Model file for the job. Use its own axes, mm. Face numbers are marked on the shaded views. A direction names the side the tool comes from. Coordinates: 2 decimals unless noted, no trailing zeros. Write each loop counter-clockwise with the first axis right and the second up, starting at its lowest first coordinate (ties: lowest second). Pieces come first, ordered by that corner, then holes. Notation, with made-up numbers: M 78.25,76.25 L 132.25,76.25 A21 cw 132.25,85.25 Z; hole C 59.25,-31.75 d10. An arc over 180 degrees is marked long. Put each result on its own line as item: value. Start each with the question number.
Q1. Cut at C-C (z = 14.5). Write the cut outline in (x, y), then the cut area to 3 significant figures.
Q2. Which spindle directions (+Z, -Z, +X, -X, +Y, -Y) get a long thin tool onto all of the face, cutting with end or side? Do the marked faces 1, 2 and 3. Say none if no direction does.
Q3. Pull direction Y, two halves, no side cores. Call the marked faces 4, 5 and 6: pulls with the +Y half, pulls with the -Y half, needs draft (parallel to the pull), parting line crosses it, or undercut.
Q4. Cut at A-A (z = 11). Write the cut outline in (x, y).
Q5. Drop flat-ended pins along their axis: pin 1 (10 mm diameter, centred on x = -7.5, z = 6, fed in from -Y); pin 2 (0.9 mm diameter, centred on x = 16.5, z = 0, fed in from -Y); pin 3 (12 mm diameter, centred on x = 31, z = 9, fed in from +Y); pin 4 (3 mm diameter, centred on x = 27.5, z = 10, fed in from -Y). Give the stop position or say it passes through.
Q6. Cut at B-B (x = 21.5). Give the number of separate pieces and of enclosed holes in the cut face, then the cut area to 3 significant figures.
Q7. Drill centre lines: line 1 along Y through (x, z) = (-1, 15.25); line 2 along Z through (x, y) = (33, -30); line 3 along Y through (x, z) = (0, 12). Where is each one in solid material? Low to high.
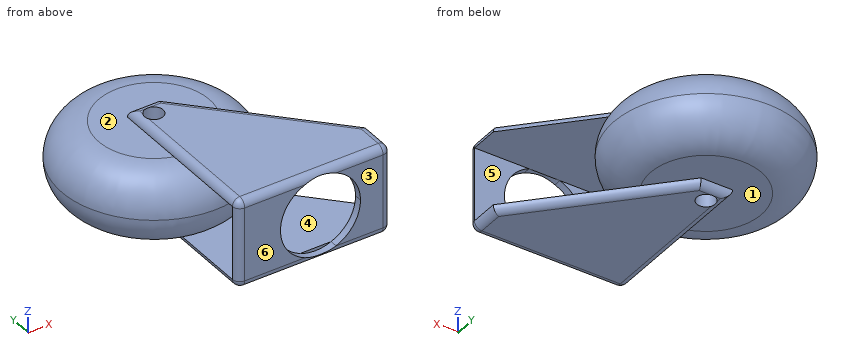
```python
from build123d import *

# Parameters (mm, degrees)
F0_R          = 25
F1_DEPTH      = 20
F2_R          = 9.99999
F3_R          = 2.5
F4_DEPTH      = 25.4
F5_R          = 2.5
F6_DEPTH      = 2
F7_W          = 41.5132804774
F7_H          = 2
F8_DEPTH      = 20
F9_R          = 2.5
F9_W          = 41.5132804774
F9_H          = 2
F10_DEPTH     = 2
F11_T1_DEPTH  = 20
F11_T3_DEPTH  = 47.4638193212
F11_T5_DEPTH  = 37.5132804774
F11_T7_DEPTH  = 12.6040666103
F11_T9_DEPTH  = 57.9730332998
F11_T11_DEPTH = 18.5555869155
F11_T13_DEPTH = 57.9730332998
F11_S17_W     = 2
F11_S17_H     = 2
F11_T18_DEPTH = 2
F11_S23_W     = 2
F11_S23_H     = 2
F11_T24_DEPTH = 2
F11_S29_W     = 2
F11_S29_H     = 2
F11_T30_DEPTH = 2
F11_S35_W     = 2
F11_S35_H     = 2
F11_T36_DEPTH = 2
F13_DEPTH     = 2


# Not quite as in the source:
# - a fillet or chamfer that OpenCascade refuses, or shapes differently, is made with other operations: its cross-section is extruded or revolved along the edge and cut away or added
# - a fillet or chamfer is up to 0.001 mm smaller than in the source, because OpenCascade refuses the exact size


with BuildPart() as f1:
    # F0 (on Top) → F1 (new body)
    with BuildSketch(Plane.XY):
        Circle(F0_R)
    extrude(amount=F1_DEPTH)

    # F2 (radius 10 in the source; OpenCascade refuses exactly that, so slightly less here)
    f2_edges = [f1.edges().sort_by_distance(p)[0] for p in [
        (-25, 0, 20),
        (-25, 0, 0),
    ]]
    fillet(f2_edges, radius=F2_R)

    # F3 (on face) → F4 (cut)
    with BuildSketch(Plane.XY.offset(20)):
        Circle(F3_R)
    extrude(amount=-F4_DEPTH, mode=Mode.SUBTRACT)

    # F5 (on face) → F6 (join)
    with BuildSketch(Plane(origin=(0, 0, 0), x_dir=(1, 0, 0), z_dir=(0, 0, -1))):
        with BuildLine():
            Line((37.3017899692, 30.3959333897), (37.3017899692, 40))
            Line((37.3017899692, 40), (-4.2114905082, 40))
            Line((-4.2114905082, 40), (-4.2114905082, 14.3966540453))
            ThreePointArc((-4.2114905082, 14.3966540453), (6.5284436355, 13.5048037268), (13.8984988304, 5.641988148))
            Line((13.8984988304, 5.641988148), (37.3017899692, 30.3959333897))
        make_face()
        with BuildLine():
            Line((4.3440964073, -4.4638193212), (13.8984988304, 5.641988148))
            ThreePointArc((13.8984988304, 5.641988148), (6.5284436355, 13.5048037268), (-4.2114905082, 14.3966540453))
            Line((-4.2114905082, 14.3966540453), (-4.2114905082, -4.4638193212))
            Line((-4.2114905082, -4.4638193212), (4.3440964073, -4.4638193212))
        make_face()
        Circle(F5_R, mode=Mode.SUBTRACT)
    extrude(amount=F6_DEPTH)

    # F7 (on face) → F8 (join)
    with BuildSketch(Plane.XY):
        with Locations((16.5451497305, -39)):
            Rectangle(F7_W, F7_H)
    extrude(amount=F8_DEPTH)

    # F9 (on face) → F10 (join)
    with BuildSketch(Plane.XY.offset(20)):
        Polygon((37.3017899692, -38), (37.3017899692, -30.3959333897), (4.3440964073, 4.4638193212), (-4.2114905082, 4.4638193212), (-4.2114905082, -38), align=None)
        Circle(F9_R, mode=Mode.SUBTRACT)
        with Locations((16.5451497305, -39)):
            Rectangle(F9_W, F9_H)
    extrude(amount=F10_DEPTH)

    # F11: fillet of radius 2 on 12 edges, made by hand

    # F11_s2 → F11_t1 (cut)
    with BuildSketch(Plane.XY):
        with BuildLine():
            ThreePointArc((-2.2114905082, -40), (-3.6257040705, -39.4142135624), (-4.2114905082, -38))
            Line((-4.2114905082, -38), (-4.2114905082, -40))
            Line((-4.2114905082, -40), (-2.2114905082, -40))
        make_face()
        with BuildLine():
            ThreePointArc((35.3017899692, -40), (36.7160035316, -39.4142135624), (37.3017899692, -38))
            Line((37.3017899692, -38), (37.3017899692, -40))
            Line((37.3017899692, -40), (35.3017899692, -40))
        make_face()
    extrude(amount=F11_T1_DEPTH, mode=Mode.SUBTRACT)

    # F11_s4 → F11_t3 (cut)
    with BuildSketch(Plane.XZ.offset(-9.4638193212)):
        with BuildLine():
            ThreePointArc((-2.2114905082, 22), (-3.6257040705, 21.4142135624), (-4.2114905082, 20))
            Line((-4.2114905082, 20), (-4.2114905082, 22))
            Line((-4.2114905082, 22), (-2.2114905082, 22))
        make_face()
        with BuildLine():
            ThreePointArc((-2.2114905082, -2), (-3.6257040705, -1.4142135624), (-4.2114905082, 0))
            Line((-4.2114905082, 0), (-4.2114905082, -2))
            Line((-4.2114905082, -2), (-2.2114905082, -2))
        make_face()
    extrude(amount=F11_T3_DEPTH, mode=Mode.SUBTRACT)

    # F11_s6 → F11_t5 (cut)
    with BuildSketch(Plane.YZ.offset(-2.2114905082)):
        with BuildLine():
            ThreePointArc((-38, 22), (-39.4142135624, 21.4142135624), (-40, 20))
            Line((-40, 20), (-40, 22))
            Line((-40, 22), (-38, 22))
        make_face()
        with BuildLine():
            ThreePointArc((-38, -2), (-39.4142135624, -1.4142135624), (-40, 0))
            Line((-40, 0), (-40, -2))
            Line((-40, -2), (-38, -2))
        make_face()
    extrude(amount=F11_T5_DEPTH, mode=Mode.SUBTRACT)

    # F11_s8 → F11_t7 (cut)
    with BuildSketch(Plane.XZ.offset(25.3959333897)):
        with BuildLine():
            ThreePointArc((35.3017899692, 22), (36.7160035316, 21.4142135624), (37.3017899692, 20))
            Line((37.3017899692, 20), (37.3017899692, 22))
            Line((37.3017899692, 22), (35.3017899692, 22))
        make_face()
        with BuildLine():
            ThreePointArc((35.3017899692, -2), (36.7160035316, -1.4142135624), (37.3017899692, 0))
            Line((37.3017899692, 0), (37.3017899692, -2))
            Line((37.3017899692, -2), (35.3017899692, -2))
        make_face()
    extrude(amount=F11_T7_DEPTH, mode=Mode.SUBTRACT)

    # F11_s10 → F11_t9 (cut)
    with BuildSketch(Plane(origin=(36.2146215396, -38.3046449843, 0), x_dir=(0, 0, 1), z_dir=(-0.6870045793, 0.7266530864, 0))):
        with BuildLine():
            ThreePointArc((20, 6.223315377), (21.4142135624, 5.6375289394), (22, 4.223315377))
            Line((22, 4.223315377), (22, 6.223315377))
            Line((22, 6.223315377), (20, 6.223315377))
        make_face()
    extrude(amount=F11_T9_DEPTH, mode=Mode.SUBTRACT)

    # F11_s12 → F11_t11 (cut)
    with BuildSketch(Plane.YZ.offset(-9.2114905082)):
        with BuildLine():
            ThreePointArc((2.4638193212, 22), (3.8780328836, 21.4142135624), (4.4638193212, 20))
            Line((4.4638193212, 20), (4.4638193212, 22))
            Line((4.4638193212, 22), (2.4638193212, 22))
        make_face()
        with BuildLine():
            ThreePointArc((2.4638193212, -2), (3.8780328836, -1.4142135624), (4.4638193212, 0))
            Line((4.4638193212, 0), (4.4638193212, -2))
            Line((4.4638193212, -2), (2.4638193212, -2))
        make_face()
    extrude(amount=F11_T11_DEPTH, mode=Mode.SUBTRACT)

    # F11_s14 → F11_t13 (cut)
    with BuildSketch(Plane(origin=(-3.6131178157, 3.8216385905, 0), x_dir=(0, 0, 1), z_dir=(0.6870045793, -0.7266530864, 0))):
        with BuildLine():
            ThreePointArc((-2, -4.223315377), (-1.4142135624, -5.6375289394), (0, -6.223315377))
            Line((0, -6.223315377), (-2, -6.223315377))
            Line((-2, -6.223315377), (-2, -4.223315377))
        make_face()
    extrude(amount=F11_T13_DEPTH, mode=Mode.SUBTRACT)


with BuildPart() as f11_tool16:
    # F11_s17 → F11_t18 (new body)
    with BuildSketch(Plane.XZ.offset(38)):
        with Locations((-3.2114905082, -1)):
            Rectangle(F11_S17_W, F11_S17_H)
    extrude(amount=F11_T18_DEPTH)

    # F11_s19 → F11_t20 (revolve, cut)
    with BuildSketch(Plane(origin=(-2.2114905082, -38, 0), x_dir=(0.7071067812, 0, 0.7071067812), z_dir=(0.7071067812, 0, -0.7071067812))):
        with BuildLine():
            ThreePointArc((0, -2), (2, 0), (0, 2))
            Line((0, 2), (0, -2))
        make_face()
    revolve(axis=Axis((-2.2114905082, -38, 0), (0, -1, 0)), mode=Mode.SUBTRACT)


with BuildPart() as f1_1:
    add(f1.part)

    # F11_t15: cut F11_tool16
    add(f11_tool16.part, mode=Mode.SUBTRACT)


with BuildPart() as f11_tool22:
    # F11_s23 → F11_t24 (new body)
    with BuildSketch(Plane.XZ.offset(38)):
        with Locations((-3.2114905082, 21)):
            Rectangle(F11_S23_W, F11_S23_H)
    extrude(amount=F11_T24_DEPTH)

    # F11_s25 → F11_t26 (revolve, cut)
    with BuildSketch(Plane(origin=(-2.2114905082, -38, 20), x_dir=(0.7071067812, 0, -0.7071067812), z_dir=(-0.7071067812, 0, -0.7071067812))):
        with BuildLine():
            ThreePointArc((0, -2), (2, 0), (0, 2))
            Line((0, 2), (0, -2))
        make_face()
    revolve(axis=Axis((-2.2114905082, -38, 20), (0, -1, 0)), mode=Mode.SUBTRACT)


with BuildPart() as f1_2:
    add(f1_1.part)

    # F11_t21: cut F11_tool22
    add(f11_tool22.part, mode=Mode.SUBTRACT)


with BuildPart() as f11_tool28:
    # F11_s29 → F11_t30 (new body)
    with BuildSketch(Plane.XZ.offset(38)):
        with Locations((36.3017899692, 21)):
            Rectangle(F11_S29_W, F11_S29_H)
    extrude(amount=F11_T30_DEPTH)

    # F11_s31 → F11_t32 (revolve, cut)
    with BuildSketch(Plane(origin=(35.3017899692, -38, 20), x_dir=(-0.7071067812, 0, -0.7071067812), z_dir=(-0.7071067812, 0, 0.7071067812))):
        with BuildLine():
            ThreePointArc((0, -2), (2, 0), (0, 2))
            Line((0, 2), (0, -2))
        make_face()
    revolve(axis=Axis((35.3017899692, -38, 20), (0, -1, 0)), mode=Mode.SUBTRACT)


with BuildPart() as f1_3:
    add(f1_2.part)

    # F11_t27: cut F11_tool28
    add(f11_tool28.part, mode=Mode.SUBTRACT)


with BuildPart() as f11_tool34:
    # F11_s35 → F11_t36 (new body)
    with BuildSketch(Plane.XZ.offset(38)):
        with Locations((36.3017899692, -1)):
            Rectangle(F11_S35_W, F11_S35_H)
    extrude(amount=F11_T36_DEPTH)

    # F11_s37 → F11_t38 (revolve, cut)
    with BuildSketch(Plane(origin=(35.3017899692, -38, 0), x_dir=(-0.7071067812, 0, 0.7071067812), z_dir=(0.7071067812, 0, 0.7071067812))):
        with BuildLine():
            ThreePointArc((0, -2), (2, 0), (0, 2))
            Line((0, 2), (0, -2))
        make_face()
    revolve(axis=Axis((35.3017899692, -38, 0), (0, -1, 0)), mode=Mode.SUBTRACT)


with BuildPart() as f1_4:
    add(f1_3.part)

    # F11_t33: cut F11_tool34
    add(f11_tool34.part, mode=Mode.SUBTRACT)

    # F12 (on face) → F13 (cut)
    with BuildSketch(Plane.XZ.offset(40)):
        with BuildLine():
            Line((14.1298108305, 20), (22.5242070351, 20))
            ThreePointArc((22.5242070351, 20), (18.3270089328, 20.8447), (14.1298108305, 20))
        make_face()
        with BuildLine():
            ThreePointArc((22.5493864515, 0), (27.3695554789, 3.9984635169), (29.1770089328, 9.9947))
            ThreePointArc((29.1770089328, 9.9947), (27.3619992319, 16.0023160243), (22.5242070351, 20))
            Line((22.5242070351, 20), (14.1298108305, 20))
            ThreePointArc((14.1298108305, 20), (7.4770175315, 10.0083598225), (14.1046314142, 0))
            Line((14.1046314142, 0), (22.5493864515, 0))
        make_face()
        with BuildLine():
            ThreePointArc((14.1046314142, 0), (18.3270089328, -0.8553), (22.5493864515, 0))
            Line((22.5493864515, 0), (14.1046314142, 0))
        make_face()
    extrude(amount=-F13_DEPTH, mode=Mode.SUBTRACT)


solid = f1_4.part
```
Computed values:
1. outline: C 0,0 d47.86; M -4.21,-38 A2 ccw -2.21,-40 L 8.46,-40 L 8.46,-38 Z; M 28.2,-40 L 35.3,-40 A2 ccw 37.3,-38 L 28.2,-38 Z; hole C 0,0 d5
1. area: 1,820 mm2
2. face 1: -Z, +Y
2. face 2: +Z, +Y
2. face 3: +Z, -Z, +X, -X, -Y
3. face 4: undercut
3. face 5: pulls with the +Y half
3. face 6: pulls with the -Y half
4. outline: C 0,0 d49.9; M -4.21,-38 A2 ccw -2.21,-40 L 7.52,-40 L 7.52,-38 Z; M 29.13,-40 L 35.3,-40 A2 ccw 37.3,-38 L 29.13,-38 Z; hole C 0,0 d5
5. pin 1: y = -39.98
5. pin 2: y = -38
5. pin 3: y = -38
5. pin 4: through
6. separate pieces: 3
6. enclosed holes: 0
6. area: 409 mm2
7. line 1: -40 to -38, -23.49 to -2.29, 2.29 to 23.49
7. line 2: -2 to 0, 20 to 22
7. line 3: -40 to -38, -24.8 to -2.5, 2.5 to 24.8
